```python
from build123d import *

# Parameters (mm, degrees)
F0_R     = 6
F1_DEPTH = 50
F2_R     = 2.5
F3_DEPTH = 25
F5_R     = 3.423218
F6_DEPTH = 25


with BuildPart() as f1:
    # F0 (on Front) → F1 (new body)
    with BuildSketch(Plane.XZ):
        with BuildLine():
            Line((0, 0), (0, 35.195496))
            Line((0, 35.195496), (-6.381311, 35.195496))
            ThreePointArc((-6.381311, 35.195496), (-8.840759, 30.764286), (-13.108497, 28.030987))
            ThreePointArc((-13.108497, 28.030987), (-20.613351, 18.062411), (-13.976716, 7.495935))
            ThreePointArc((-13.976716, 7.495935), (-9.473946, 4.46239), (-6.381311, 0))
            Line((-6.381311, 0), (0, 0))
        make_face()
        with Locations((-9.623169, 17.597748)):
            Circle(F0_R, mode=Mode.SUBTRACT)
    extrude(amount=F1_DEPTH)

    # F2 (on face) → F3 (cut)
    with BuildSketch(Plane.YZ):
        with Locations((-39, 29.195496)):
            Circle(F2_R)
        with Locations((-11, 29.195496)):
            Circle(F2_R)
        with Locations((-39, 6)):
            Circle(F2_R)
        with Locations((-11, 6)):
            Circle(F2_R)
    extrude(amount=-F3_DEPTH, mode=Mode.SUBTRACT)

    # F5 (on offset) → F6 (cut)
    with BuildSketch(Plane.YZ.offset(-6.5)):
        with Locations((-11, 6)):
            Circle(F5_R)
        with Locations((-39, 6)):
            Circle(F5_R)
        with Locations((-11, 29.195496)):
            Circle(F5_R)
        with Locations((-39, 29.195496)):
            Circle(F5_R)
    extrude(amount=-F6_DEPTH, mode=Mode.SUBTRACT)


solid = f1.part
```
Part model, mm, in its own coordinate system. A direction names the side the tool comes from. Give positions to 0.01 mm unless a question says otherwise; leave off trailing zeros. Write each loop counter-clockwise with the first axis right and the second up, starting at its lowest first coordinate (ties: lowest second). Pieces come first, ordered by that corner, then holes. Notation, with made-up numbers: (29, 77) -> (61, 77) arc R26 cw to (61, 116) -> close; hole circle Ø10 at (85, 20.5). An arc over 180 degrees is marked (long way). Put each result on its own line as item: value. Start each with the question number.
Item 1: Cut at B-B (y = -39). List the corners of the cut face in (x, z).
Item 2: Cut at D-D (y = -6.5). List the corners of the cut face in (x, z).
Item 3: Pin check, flat tips, straight feed: pin 1 Ø3 at (y, z) = (-20, 31.5) entering from -X; pin 2 Ø1.5 at (x, y) = (-9.5, -17) entering from -Z. Stop position of each tip, or through.
Item 4: Cut at A-A (x = -4.25). List the corners of the cut face in (y, z), then the cut area to 3 significant figures.
Item 5: Wall check: L1, parallel to Z at x = -2, y = -39; L2, parallel to Y at x = -10.75, z = 6; L3, parallel to X at y = -3.5, z = 17.5. Give the ranges that are in metal, low to high. Write a range as [from, to].
Item 6: Pull direction Z, two halves, no side cores. Call faces 1 (the face through (-8.696, -24.65, 3.633)), 2 (the face through (-6.5, -39, 3)), 3 (the face through (0, -25, 17)): pulls with the +Z half, pulls with the -Z half, needs draft (parallel to the pull), parting line crosses it, or undercut.
Item 7: Which spindle directions (+Z, -Z, +X, -X, +Y, -Y) get a long thin tool onto all of the face, cutting with end or side? Do faces 4 (the face through (-6.5, -41, 27)), 5 (the face through (-3.204, -36.615, 6.751)). Say none if no direction does.
Item 8: Cut at C-C (z = 6). List the corners of the cut face in (x, y), then the cut area to 3 significant figures.
Answer list:
1. outline: (-16.98, 9.42) -> (-6.5, 9.42) -> (-6.5, 8.5) -> (0, 8.5) -> (0, 26.7) -> (-6.5, 26.7) -> (-6.5, 25.77) -> (-16.98, 25.77) arc R11 ccw to start; (-7.86, 2.58) arc R14.68 cw to (-6.38, 0) -> (0, 0) -> (0, 3.5) -> (-6.5, 3.5) -> (-6.5, 2.58) -> close; (-7.45, 32.62) -> (-6.5, 32.62) -> (-6.5, 31.7) -> (0, 31.7) -> (0, 35.2) -> (-6.38, 35.2) arc R10.35 cw to start; hole circle Ø12 at (-9.62, 17.6)
2. outline: (-13.98, 7.5) arc R14.68 cw to (-6.38, 0) -> (0, 0) -> (0, 35.2) -> (-6.38, 35.2) arc R10.35 cw to (-13.11, 28.03) arc R11 ccw to start; hole circle Ø12 at (-9.62, 17.6)
3. pin 1: stops at x = -9.64
3. pin 2: stops at z = 3.69
4. outline: (-50, 0) -> (0, 0) -> (0, 14.93) -> (-50, 14.93) -> close; (-50, 20.27) -> (0, 20.27) -> (0, 35.2) -> (-50, 35.2) -> close; hole circle Ø5 at (-39, 6); hole circle Ø5 at (-39, 29.2); hole circle Ø5 at (-11, 6); hole circle Ø5 at (-11, 29.2)
4. area: 1,410 mm2
5. L1: z = [0, 3.5], [8.5, 26.7], [31.7, 35.2]
5. L2: y = [-50, -42.42], [-35.58, -14.42], [-7.58, 0]
5. L3: x = [-20.62, -15.62], [-3.62, 0]
6. face 1: pulls with the -Z half
6. face 2: undercut
6. face 3: needs draft
7. face 4: -X
7. face 5: +X, -X
8. outline: (-11.31, -50) -> (0, -50) -> (0, -41.5) -> (-6.5, -41.5) -> (-6.5, -42.42) -> (-11.31, -42.42) -> close; (-11.31, -35.58) -> (-6.5, -35.58) -> (-6.5, -36.5) -> (0, -36.5) -> (0, -13.5) -> (-6.5, -13.5) -> (-6.5, -14.42) -> (-11.31, -14.42) -> close; (-11.31, -7.58) -> (-6.5, -7.58) -> (-6.5, -8.5) -> (0, -8.5) -> (0, 0) -> (-11.31, 0) -> close
8. area: 435 mm2
